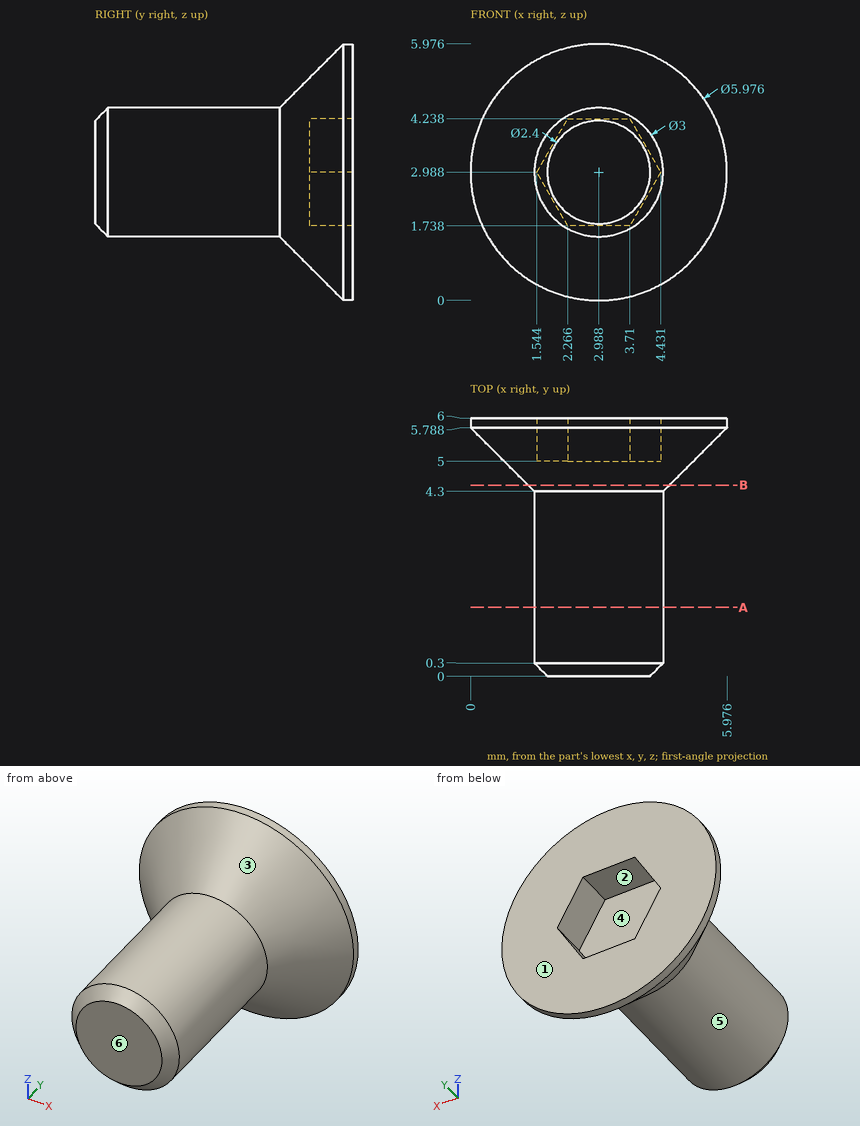
The drawing under review shows one solid part. Ordinate dimensions are in mm from its lowest x, y, z. A direction names the side the tool comes from. Round coordinates to 2 decimals unless told otherwise and drop trailing zeros. Write each loop counter-clockwise with the first axis right and the second up, starting at its lowest first coordinate (ties: lowest second). Pieces come first, ordered by that corner, then holes. Notation, with made-up numbers: (-31, 75) -> (-23, 75) arc R28 cw to (-23, 105) -> close; hole circle Ø6 at (48, -17.75). An arc over 180 degrees is marked (long way). One line per question, with ' | ' between items.
(1) Machinability: for the marked faces 4, 5 and 6, which of the approach directions +Z, -Z, +X, -X, +Y, -Y give a long, thin tool a straight path to every point of the face, cutting with its end or side? Answer none if there is none.
Result sheet:
face 4: +Y | face 5: -Y | face 6: +Z, -Z, +X, -X, -Y
(2) Draft analysis for pull direction Z (two halves, no side actions). For the marked faces 1, 2 and 3, state which applies: released by +Z, released by -Z, zero draft, split by the parting line, or undercut.
Result sheet:
face 1: zero draft | face 2: undercut | face 3: split by the parting line
(3) Insertion check: P1, Ø1, axis at y = 3, z = 1.5, coming from the +X side (1 decimal); P2, Ø1.2, axis at x = 3.5, z = 3, coming from the +Y side; P3, Ø1.5, axis at y = 5, z = 0.5, coming from the -X side (1 decimal). Each pin has a flat end and moves straight along its axis. Give the tip position at first contact, or say it passes through.
Result sheet:
P1: x = 4.1 | P2: y = 5 | P3: x = 1.1
(4) Take a section at B-B, the plane y = 4.45. State the section outline as (x, z) points.
Result sheet:
outline: circle Ø3.3 at (2.99, 2.99)
(5) Take a section at A-A, the plane y = 1.6. State the section outline as (x, z) points.
Result sheet:
outline: circle Ø3 at (2.99, 2.99)
(6) Wall thickness on line 1 (Z direction, x = 1.6, y = 5.6) (1 decimal); line 2 (X direction, y = 5.15, z = 1) (1 decimal); line 3 (Z direction, x = 2.8, y = 1.55) (1 decimal): over which ranges is each line inside the solid? List them lowest first. Write a range as [from, to].
Result sheet:
line 1: [0.6, 2.9], [3.1, 5.4] | line 2: [1.7, 4.2] | line 3: [1.5, 4.5]
